```python
from build123d import *

# Parameters (mm, degrees)
SKETCH1_R           = 21.59
BOSS_EXTRUDE1_DEPTH = 6.35
SKETCH2_R           = 4.572
CUT_EXTRUDE1_DEPTH  = 7.35
SKETCH3_R           = 2.54
SKETCH3_R_2         = 7.62
SKETCH3_R_3         = 4.572
CUT_EXTRUDE2_DEPTH  = 3.175
SKETCH4_R           = 2.54
SKETCH4_R_2         = 7.62
SKETCH4_R_3         = 4.572
BOSS_EXTRUDE2_DEPTH = 1.27


with BuildPart() as part:
    # Sketch1 → Boss-Extrude1 (new body)
    with BuildSketch(Plane(origin=(0, 0, 0), x_dir=(1, 0, 0), z_dir=(0, 1, 0))):
        Circle(SKETCH1_R)
    extrude(amount=BOSS_EXTRUDE1_DEPTH)

    # Sketch2 → Cut-Extrude1 (cut, through all)
    with BuildSketch(Plane.XZ):
        Circle(SKETCH2_R)
    extrude(amount=-CUT_EXTRUDE1_DEPTH, mode=Mode.SUBTRACT)

    # Sketch3 → Cut-Extrude2 (cut)
    with BuildSketch(Plane.XZ):
        with BuildLine():
            ThreePointArc((4.587624646, -6.084250168), (0, -7.62), (-4.587624646, -6.084250168))
            Line((-4.587624646, -6.084250168), (-4.318, -7.62))
            Line((-4.318, -7.62), (-2.5017368, -17.965218605))
            ThreePointArc((-2.5017368, -17.965218605), (-0.220441067, -14.995583881), (2.54, -17.526))
            ThreePointArc((2.54, -17.526), (2.530416119, -17.746441067), (2.5017368, -17.965218605))
            Line((2.5017368, -17.965218605), (4.318, -7.62))
            Line((4.318, -7.62), (4.587624646, -6.084250168))
        make_face()
        with Locations((0, -17.526)):
            Circle(SKETCH3_R)
        with BuildLine():
            Line((-17.965218605, -2.5017368), (-7.62, -4.318))
            Line((-7.62, -4.318), (-6.084250168, -4.587624646))
            ThreePointArc((-6.084250168, -4.587624646), (-7.62, 0), (-6.084250168, 4.587624646))
            Line((-6.084250168, 4.587624646), (-7.62, 4.318))
            Line((-7.62, 4.318), (-17.965218605, 2.5017368))
            ThreePointArc((-17.965218605, 2.5017368), (-15.892600976, 1.94514977), (-14.986, 0))
            ThreePointArc((-14.986, 0), (-15.892600976, -1.94514977), (-17.965218605, -2.5017368))
        make_face()
        with Locations((-17.526, 0)):
            Circle(SKETCH3_R)
        Circle(SKETCH3_R_2)
        Circle(SKETCH3_R_3, mode=Mode.SUBTRACT)
        with BuildLine():
            Line((-4.318, 7.62), (-4.587624646, 6.084250168))
            ThreePointArc((-4.587624646, 6.084250168), (0, 7.62), (4.587624646, 6.084250168))
            Line((4.587624646, 6.084250168), (4.318, 7.62))
            Line((4.318, 7.62), (2.5017368, 17.965218605))
            ThreePointArc((2.5017368, 17.965218605), (2.530416119, 17.746441067), (2.54, 17.526))
            ThreePointArc((2.54, 17.526), (-0.220441067, 14.995583881), (-2.5017368, 17.965218605))
            Line((-2.5017368, 17.965218605), (-4.318, 7.62))
        make_face()
        with Locations((0, 17.526)):
            Circle(SKETCH3_R)
        with Locations((17.526, 0)):
            Circle(SKETCH3_R)
        with BuildLine():
            ThreePointArc((7.62, 0), (7.225869715, -2.418926799), (6.084250168, -4.587624646))
            Line((6.084250168, -4.587624646), (7.62, -4.318))
            Line((7.62, -4.318), (17.965218605, -2.5017368))
            ThreePointArc((17.965218605, -2.5017368), (14.986, 0), (17.965218605, 2.5017368))
            Line((17.965218605, 2.5017368), (7.62, 4.318))
            Line((7.62, 4.318), (6.084250168, 4.587624646))
            ThreePointArc((6.084250168, 4.587624646), (7.225869715, 2.418926799), (7.62, 0))
        make_face()
    extrude(amount=-CUT_EXTRUDE2_DEPTH, mode=Mode.SUBTRACT)

    # Sketch4 → Boss-Extrude2 (add)
    with BuildSketch(Plane(origin=(0, 6.35, 0), x_dir=(1, 0, 0), z_dir=(0, 1, 0))):
        with BuildLine():
            Line((4.318, 7.62), (2.5017368, 17.965218605))
            ThreePointArc((2.5017368, 17.965218605), (2.530416119, 17.746441067), (2.54, 17.526))
            ThreePointArc((2.54, 17.526), (-0.220441067, 14.995583881), (-2.5017368, 17.965218605))
            Line((-2.5017368, 17.965218605), (-4.318, 7.62))
            Line((-4.318, 7.62), (-4.587624646, 6.084250168))
            ThreePointArc((-4.587624646, 6.084250168), (0, 7.62), (4.587624646, 6.084250168))
            Line((4.587624646, 6.084250168), (4.318, 7.62))
        make_face()
        with Locations((0, 17.526)):
            Circle(SKETCH4_R)
        with BuildLine():
            Line((-7.62, -4.318), (-6.084250168, -4.587624646))
            ThreePointArc((-6.084250168, -4.587624646), (-7.62, 0), (-6.084250168, 4.587624646))
            Line((-6.084250168, 4.587624646), (-7.62, 4.318))
            Line((-7.62, 4.318), (-17.965218605, 2.5017368))
            ThreePointArc((-17.965218605, 2.5017368), (-15.892600976, 1.94514977), (-14.986, 0))
            ThreePointArc((-14.986, 0), (-15.892600976, -1.94514977), (-17.965218605, -2.5017368))
            Line((-17.965218605, -2.5017368), (-7.62, -4.318))
        make_face()
        with Locations((-17.526, 0)):
            Circle(SKETCH4_R)
        with Locations((0, -17.526)):
            Circle(SKETCH4_R)
        with BuildLine():
            Line((2.5017368, -17.965218605), (4.318, -7.62))
            Line((4.318, -7.62), (4.587624646, -6.084250168))
            ThreePointArc((4.587624646, -6.084250168), (0, -7.62), (-4.587624646, -6.084250168))
            Line((-4.587624646, -6.084250168), (-4.318, -7.62))
            Line((-4.318, -7.62), (-2.5017368, -17.965218605))
            ThreePointArc((-2.5017368, -17.965218605), (-0.220441067, -14.995583881), (2.54, -17.526))
            ThreePointArc((2.54, -17.526), (2.530416119, -17.746441067), (2.5017368, -17.965218605))
        make_face()
        with BuildLine():
            ThreePointArc((7.62, 0), (7.225869715, -2.418926799), (6.084250168, -4.587624646))
            Line((6.084250168, -4.587624646), (7.62, -4.318))
            Line((7.62, -4.318), (17.965218605, -2.5017368))
            ThreePointArc((17.965218605, -2.5017368), (14.986, 0), (17.965218605, 2.5017368))
            Line((17.965218605, 2.5017368), (7.62, 4.318))
            Line((7.62, 4.318), (6.084250168, 4.587624646))
            ThreePointArc((6.084250168, 4.587624646), (7.225869715, 2.418926799), (7.62, 0))
        make_face()
        with Locations((17.526, 0)):
            Circle(SKETCH4_R)
        Circle(SKETCH4_R_2)
        Circle(SKETCH4_R_3, mode=Mode.SUBTRACT)
    extrude(amount=BOSS_EXTRUDE2_DEPTH)


solid = part.part
```
Could you check a few things on this model? Use its own coordinates, in mm. A direction names the side the tool comes from. Coordinates: 2 decimals unless noted, no trailing zeros. Loops run counter-clockwise (first coordinate to the right, second up) from the corner with the lowest first, then second, coordinate; pieces in that order, holes last.
1) Imagine slicing it at C-C (x = 0). List the corners of the cut face in (y, z) for me (3 decimals).
Reported:
outline: (0, -21.59) - (6.35, -21.59) - (6.35, -20.066) - (7.62, -20.066) - (7.62, -4.572) - (3.175, -4.572) - (3.175, -20.066) - (0, -20.066) - close; (0, 20.066) - (3.175, 20.066) - (3.175, 4.572) - (7.62, 4.572) - (7.62, 20.066) - (6.35, 20.066) - (6.35, 21.59) - (0, 21.59) - close
2) Imagine slicing it at A-A (z = 0). List the corners of the cut face in (x, y) for me (3 decimals).
Reported:
outline: (-21.59, 0) - (-20.066, 0) - (-20.066, 3.175) - (-4.572, 3.175) - (-4.572, 7.62) - (-20.066, 7.62) - (-20.066, 6.35) - (-21.59, 6.35) - close; (4.572, 3.175) - (20.066, 3.175) - (20.066, 0) - (21.59, 0) - (21.59, 6.35) - (20.066, 6.35) - (20.066, 7.62) - (4.572, 7.62) - close
3) Imagine slicing it at B-B (y = 2). List the corners of the cut face in (x, z) for me.
Reported:
outline: circle Ø43.18 at (0, 0); hole (-17.97, -2.5) - (-6.08, -4.59) arc R7.62 ccw to (-4.59, -6.08) - (-2.5, -17.97) arc R2.54 ccw to (2.5, -17.97) - (4.59, -6.08) arc R7.62 ccw to (6.08, -4.59) - (17.97, -2.5) arc R2.54 ccw to (17.97, 2.5) - (6.08, 4.59) arc R7.62 ccw to (4.59, 6.08) - (2.5, 17.97) arc R2.54 ccw to (-2.5, 17.97) - (-4.59, 6.08) arc R7.62 ccw to (-6.08, 4.59) - (-17.97, 2.5) arc R2.54 ccw to start
4) Please list where these lines run through material, in increasing order: line 1 along X through (y, z) = (5.35, 0); line 2 along Y through (x, z) = (-10, -4).
Reported:
line 1: x = -21.59 to -4.57, 4.57 to 21.59
line 2: y = 0 to 6.35
5) Imagine slicing it at D-D (z = -16). List the corners of the cut face in (x, y) for me (3 decimals).
Reported:
outline: (-14.496, 0) - (-2.847, 0) - (-2.847, 3.175) - (2.847, 3.175) - (2.847, 0) - (14.496, 0) - (14.496, 6.35) - (2.847, 6.35) - (2.847, 7.62) - (-2.847, 7.62) - (-2.847, 6.35) - (-14.496, 6.35) - close
6) Will these pins go through, and if not, where does the flat tip stop? pin 1 Ø1 at (x, y) = (13, 5.5) entering from +Z; pin 2 Ø2 at (x, y) = (-8.5, 1.5) entering from -Z; pin 3 Ø4 at (x, y) = (-5, 3.5) entering from -Z; pin 4 Ø8 at (x, z) = (0, 0) entering from +Y.
Reported:
pin 1: stops at z = 17.6
pin 2: stops at z = -20.25
pin 3: stops at z = -21.38
pin 4: passes through
7) Thinking about a two-plate mould opening in Z: for faces 6 (the face through (5.378, 6.976, 5.399)), 7 (the face through (20.066, 1.565, -0.05)), 8 (the face through (9.3, 6.35, 4.5)), 9 (the face through (0.05, 6.976, -20.066)), which applies, released by +Z, released by -Z, zero draft, split by the parting line, or undercut?
Reported:
face 6: released by +Z
face 7: undercut
face 8: zero draft
face 9: released by -Z
8) Which directions (+Z, -Z, +X, -X, +Y, -Y) give clear straight access to the entire face, cutting with the end or side of a thin tool? Please do faces 1 (the face through (-0.05, 6.976, 20.066)), 2 (the face through (-5.399, 6.976, 5.378)), 3 (the face through (20.066, 6.976, 0.05)), 4 (the face through (-20.066, 6.976, -0.05)), 5 (the face through (0.05, 1.565, 20.066)).
Reported:
face 1: +Z, +Y
face 2: +Z, -X, +Y
face 3: +X, +Y
face 4: -X, +Y
face 5: -Y
